Job drawing, mm, ordinate dimensions from the low corner. One solid piece. Coordinates: 2 decimals unless noted, no trailing zeros. Order: outer loops, then holes, each group sorted by start corner. A loop starts at its lowest first (then second) coordinate and runs counter-clockwise, first axis right, second up. Notation, with made-up numbers: (76.5, -29.75) - (121.5, -29.75) arc R32 cw to (121.5, -0.75) - close; hole circle Ø8 at (-20, -29). An arc over 180 degrees is marked (long way). Return JSON: item names as keys, results as strings.
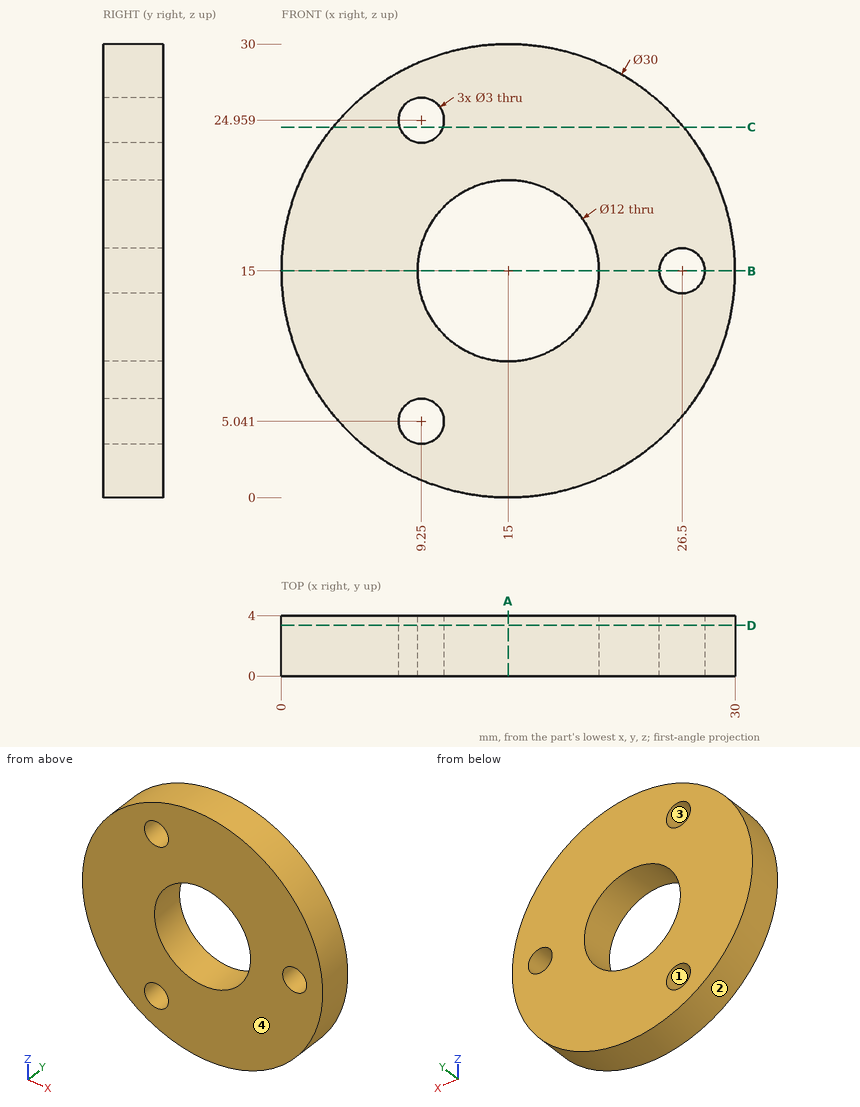
1. Cut at D-D on y = 3.35. Give the cut face in (x, z).
Check values:
{"outline": "circle Ø30 at (15, 15); hole circle Ø3 at (9.25, 5.04); hole circle Ø3 at (9.25, 24.96); hole circle Ø12 at (15, 15); hole circle Ø3 at (26.5, 15)"}
2. Cut at B-B on z = 15. Give the cut face in (x, y), plus the area to 3 significant figures.
Check values:
{"outline": "(0, 0) - (9, 0) - (9, 4) - (0, 4) - close; (21, 0) - (25, 0) - (25, 4) - (21, 4) - close; (28, 0) - (30, 0) - (30, 4) - (28, 4) - close", "area": "60.0 mm²"}
3. Cut at A-A on x = 15. Give the cut face in (y, z), plus the area to 3 significant figures.
Check values:
{"outline": "(0, 0) - (4, 0) - (4, 9) - (0, 9) - close; (0, 21) - (4, 21) - (4, 30) - (0, 30) - close", "area": "72.0 mm²"}
4. Probe L1, parallel to X at y = 3.15, z = 15; L2, parallel to Z at x = 15, y = 2; L3, parallel to Z at x = 26.5, y = 1.5. List the from-to ranges inside material, lowest first.
Check values:
{"L1": "0 to 9, 21 to 25, 28 to 30", "L2": "0 to 9, 21 to 30", "L3": "5.37 to 13.5, 16.5 to 24.63"}
5. Drop flat-ended pins along their axis: pin 1 (1 mm diameter, centred on x = 9, y = 3, fed in from -Z) (1 decimal); pin 2 (2.5 mm diameter, centred on x = 9.25, z = 24.96, fed in from +Y); pin 3 (1 mm diameter, centred on x = 25, y = 1, fed in from -Z); pin 4 (3 mm diameter, centred on x = 9, z = 12, fed in from -Y). Give the stop position or say it passes through.
Check values:
{"pin 1": "z = 1", "pin 2": "through", "pin 3": "z = 3.39", "pin 4": "y = 0"}
6. Cut at C-C on z = 24.5. Give the cut face in (x, y).
Check values:
{"outline": "(3.39, 0) - (7.82, 0) - (7.82, 4) - (3.39, 4) - close; (10.68, 0) - (26.61, 0) - (26.61, 4) - (10.68, 4) - close"}
7. Mould opens along X. For the marked faces 1, 2, 3 and 4 say: pulls with the +X half, pulls with the -X half, needs draft (parallel to the pull), parting line crosses it, or undercut.
Check values:
{"face 1": "undercut", "face 2": "parting line crosses it", "face 3": "undercut", "face 4": "needs draft"}
